Work out the finished part from the listing and answer in its coordinate system (mm). Face numbers are marked on the shaded views. A direction names the side the tool comes from. Coordinates: 2 decimals unless noted, no trailing zeros. Loops run counter-clockwise (first coordinate to the right, second up) from the corner with the lowest first, then second, coordinate; pieces in that order, holes last. Notation, with made-up numbers: (-4.75, -16.5) - (34.25, -16.5) arc R33 ccw to (34.25, 22.5) - close; hole circle Ø5 at (-19, -35). An arc over 180 degrees is marked (long way). Write each question's results on one line, items separated by ' | '. Start each with the question number.
1. Find the intervals of material crossed by line 1 along X through (y, z) = (1.05, -30); line 2 along Z through (x, y) = (58.5, 1.1); line 3 along Z through (x, y) = (45.5, 4.75), in increasing order. Write a range as [from, to].
2. A cutting plane is placed at A-A on x = 58.5. Determine the outline of the cut face in (y, z).
3. A cutting plane is placed at D-D on x = -58.5. Determine the outline of the cut face in (y, z), then the cut area to 3 significant figures.
4. Determine the mould class of the marked faces 4, 5, 6 and 7 for opening direction X: released by +X, released by -X, zero draft, split by the parting line, or undercut.
5. A cutting plane is placed at C-C on x = 27.5. Determine the outline of the cut face in (y, z).
6. Each of these flat-tipped pins is pushed along its axis until it touches: P1, Ø4, axis at y = 4.5, z = 33, coming from the +X side; P2, Ø1.5, axis at y = 3, z = 29.5, coming from the -X side; P3, Ø3, axis at y = 2.5, z = 33, coming from the -X side; P4, Ø10, axis at x = 1.5, z = 32, coming from the +Y side. Where does it stop, or does it pass through?
7. Which of the six approach directions +Z, -Z, +X, -X, +Y, -Y give full straight-line access (tool end or side, diameter ignored) to the marked faces 1, 2 and 3?
8. A cutting plane is placed at B-B on z = -30. Determine the outline of the cut face in (x, y).
from build123d import *

# Parameters (mm, degrees)
ESQUISSE1_W        = 127
ESQUISSE1_H        = 70
ESQUISSE1_R        = 1.5
BOSS_EXTRU_1_DEPTH = 1.5
ESQUISSE2_W        = 16
ESQUISSE2_H        = 9
BOSS_EXTRU_2_DEPTH = 2.5
ESQUISSE2_3_W      = 16
ESQUISSE2_3_H      = 9
BOSS_EXTRU_3_DEPTH = 5
ESQUISSE2_4_W      = 21.5
ESQUISSE2_4_H      = 16.5
ESQUISSE2_4_W_2    = 4
BOSS_EXTRU_4_DEPTH = 19


with BuildPart() as part:
    # Esquisse1 → Boss.-Extru.1 (new body)
    with BuildSketch(Plane(origin=(0, 0, 0), x_dir=(1, 0, 0), z_dir=(0, 1, 0))):
        Rectangle(ESQUISSE1_W, ESQUISSE1_H)
        with Locations((-58.5, 30)):
            Circle(ESQUISSE1_R, mode=Mode.SUBTRACT)
        with Locations((-58.5, -30)):
            Circle(ESQUISSE1_R, mode=Mode.SUBTRACT)
        with Locations((58.5, 30)):
            Circle(ESQUISSE1_R, mode=Mode.SUBTRACT)
        with Locations((58.5, -30)):
            Circle(ESQUISSE1_R, mode=Mode.SUBTRACT)
    extrude(amount=BOSS_EXTRU_1_DEPTH)

    # Esquisse2 → Boss.-Extru.2 (add)
    with BuildSketch(Plane(origin=(0, 1.5, 0), x_dir=(1, 0, 0), z_dir=(0, 1, 0))):
        with Locations((-46.3, -31.5)):
            Rectangle(ESQUISSE2_W, ESQUISSE2_H)
        with Locations((22.7, -31.5)):
            Rectangle(ESQUISSE2_W, ESQUISSE2_H)
    extrude(amount=BOSS_EXTRU_2_DEPTH)

    # Esquisse2_3 → Boss.-Extru.3 (add)
    with BuildSketch(Plane(origin=(0, 1.5, 0), x_dir=(1, 0, 0), z_dir=(0, 1, 0))):
        with Locations((-23.3, -31.5)):
            Rectangle(ESQUISSE2_3_W, ESQUISSE2_3_H)
        with Locations((-0.3, -31.5)):
            Rectangle(ESQUISSE2_3_W, ESQUISSE2_3_H)
        with Locations((45.7, -31.5)):
            Rectangle(ESQUISSE2_3_W, ESQUISSE2_3_H)
    extrude(amount=BOSS_EXTRU_3_DEPTH)

    # Esquisse2_4 → Boss.-Extru.4 (add)
    with BuildSketch(Plane(origin=(0, 1.5, 0), x_dir=(1, 0, 0), z_dir=(0, 1, 0))):
        with Locations((52.75, -3.25)):
            Rectangle(ESQUISSE2_4_W, ESQUISSE2_4_H)
        with Locations((65.5, -3.25)):
            Rectangle(ESQUISSE2_4_W_2, ESQUISSE2_4_H)
    extrude(amount=BOSS_EXTRU_4_DEPTH)


solid = part.part
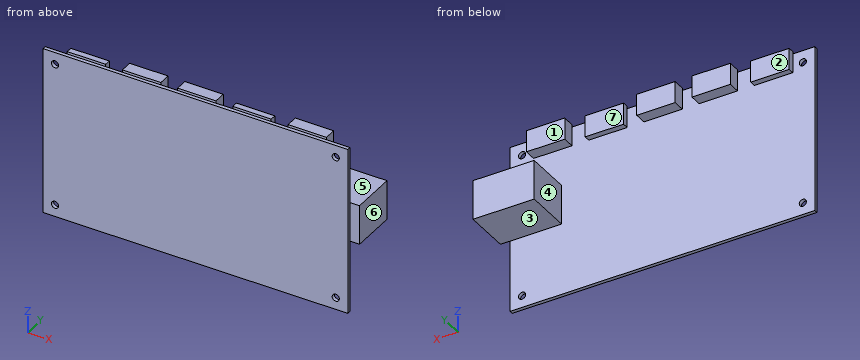
Values:
1) line 1: [-63.5, -60], [-57, 57], [60, 63.5] | line 2: [-35, -31.5], [-28.5, 28.5], [31.5, 35] | line 3: [-5, 11.5], [27, 36]
2) outline: (0, -35) - (1.5, -35) - (1.5, -31.5) - (0, -31.5) - close; (0, -28.5) - (1.5, -28.5) - (1.5, -5) - (20.5, -5) - (20.5, 11.5) - (1.5, 11.5) - (1.5, 28.5) - (0, 28.5) - close; (0, 31.5) - (1.5, 31.5) - (1.5, 35) - (0, 35) - close
3) outline: (0, -35) - (1.5, -35) - (1.5, -31.5) - (0, -31.5) - close; (0, -28.5) - (1.5, -28.5) - (1.5, 28.5) - (0, 28.5) - close; (0, 31.5) - (1.5, 31.5) - (1.5, 35) - (0, 35) - close | area: 96.0 mm^2
4) face 4: released by -X | face 5: zero draft | face 6: released by +X | face 7: undercut
5) outline: (0, -35) - (1.5, -35) - (1.5, 27) - (4, 27) - (4, 36) - (1.5, 36) - (1.5, 35) - (0, 35) - close
6) P1: x = 53.7 | P2: x = -54.3 | P3: x = -63.5 | P4: y = 6.5
7) face 1: +Z, +X, -X, +Y | face 2: +Z, -Z, -X, +Y | face 3: -Z, +X, -X, +Y
8) outline: (-63.5, 0) - (-60, 0) - (-60, 1.5) - (-63.5, 1.5) - close; (-57, 0) - (57, 0) - (57, 1.5) - (-57, 1.5) - close; (60, 0) - (63.5, 0) - (63.5, 1.5) - (60, 1.5) - close
